Could you check a few things on this drawing? It's one solid part, dimensions in mm from its lowest x, y, z. A direction names the side the tool comes from. Give positions to 0.01 mm unless a question says otherwise; leave off trailing zeros. Loops run counter-clockwise (first coordinate to the right, second up) from the corner with the lowest first, then second, coordinate; pieces in that order, holes last. Notation, with made-up numbers: M -29.75,-32 L -24.75,-32 A22 ccw -24.75,-13 Z; hole C 86,81.25 d1. An arc over 180 degrees is marked long. Return JSON: item names as keys, results as strings. Group by question number.
1. For the marked faces 1, 2 and 3, which set-ups out of +Z, -Z, +X, -X, +Y, -Y let a thin tool reach every point of the face, with its end or its side?
2. Please list where these lines run through material, in increasing order: line 1 (Z direction, x = 308, y = 133.5); line 2 (X direction, y = 44.5, z = 77) (1 decimal); line 3 (X direction, y = 102, z = 95).
3. If we section it at A-A (y = 45): Write out the boundary of the cut face in (x, z), plus the area to 3 significant figures.
4. If we section it at C-C (x = 350): Write out the boundary of the cut face in (y, z), plus the area to 3 significant figures.
5. If we section it at B-B (z = 80): Write out the boundary of the cut face in (x, y), plus the area to 3 significant figures.
6. For pin 1 (5 mm diameter, centred on y = 110.5, z = 60, fed in from -X); pin 2 (3 mm diameter, centred on y = 65.5, z = 11, fed in from -X); pin 3 (21 mm diameter, centred on y = 39.5, z = 77.5, fed in from +X), each with a flat end and sliding along its axis, tell me the tip position at first contact or that it passes through.
7. If we section it at D-D (x = 190.5): Write out the boundary of the cut face in (y, z), plus the area to 3 significant figures.
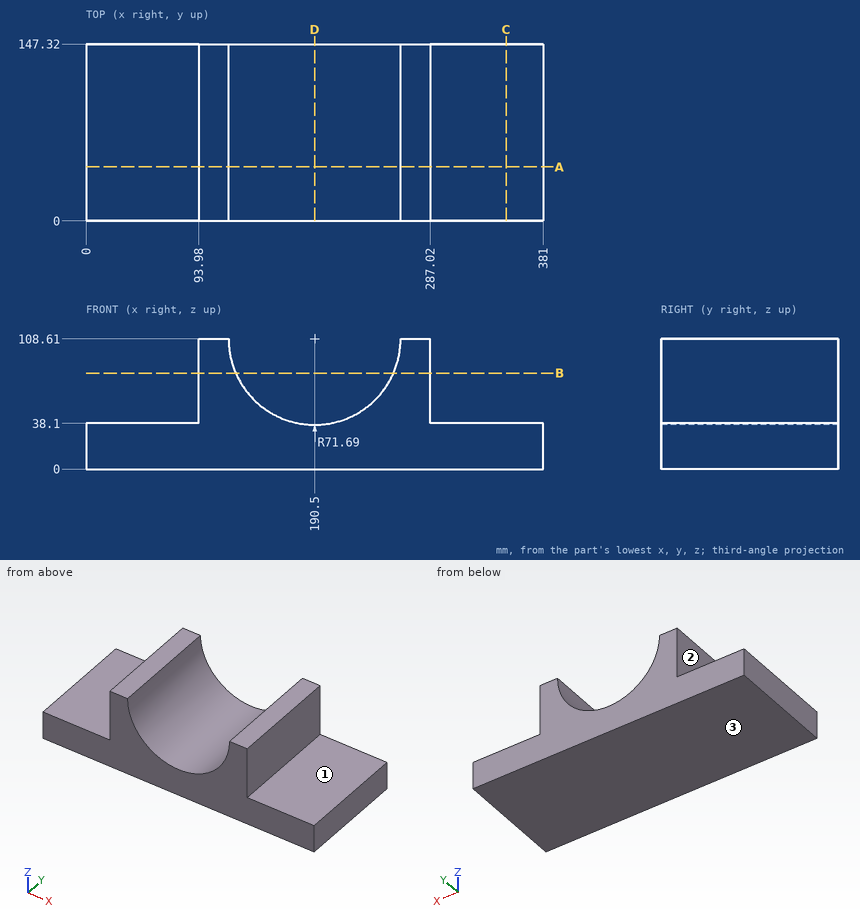
Answer:
{
 "1": {"face 1": "+Z, +X, +Y, -Y", "face 2": "+Z, -X, +Y, -Y", "face 3": "-Z, +X, -X, +Y, -Y"},
 "2": {"line 1": "z = 0 to 38.1", "line 2": "x = 94 to 126.2, 254.8 to 287", "line 3": "x = 93.98 to 120.11, 260.89 to 287.02"},
 "3": {"outline": "M 0,0 L 381,0 L 381,38.1 L 287.02,38.1 L 287.02,108.61 L 262.19,108.61 A71.69 cw 118.81,108.61 L 93.98,108.61 L 93.98,38.1 L 0,38.1 Z", "area": "20,100 mm²"},
 "4": {"outline": "M 0,0 L 147.32,0 L 147.32,38.1 L 0,38.1 Z", "area": "5,610 mm²"},
 "5": {"outline": "M 93.98,0 L 124.77,0 L 124.77,147.32 L 93.98,147.32 Z; M 256.23,0 L 287.02,0 L 287.02,147.32 L 256.23,147.32 Z", "area": "9,070 mm²"},
 "6": {"pin 1": "stops at x = 93.98", "pin 2": "stops at x = 0", "pin 3": "stops at x = 287.02"},
 "7": {"outline": "M 0,0 L 147.32,0 L 147.32,36.92 L 0,36.92 Z", "area": "5,440 mm²"}
}
